from build123d import *
from build123d.topology import SkipClean

# Parameters (mm, degrees)
SKETCH1_R                      = 10.75
SKETCH1_R_2                    = 1.25
BOSS_EXTRUDE1_DEPTH            = 12
SKETCH14_R                     = 3.25
CUT_EXTRUDE3_DEPTH             = 2.3
CBORE_FOR_M3_SHCS2_D           = 3.4
CBORE_FOR_M3_SHCS2_CBORE_D     = 6.5
CBORE_FOR_M3_SHCS2_CBORE_DEPTH = 3
SKETCH3_R                      = 9.965776233
BOSS_EXTRUDE2_DEPTH            = 20
CUT_EXTRUDE2_REACH             = 37.428
CUT_EXTRUDE1_DEPTH             = 26.122201337
CUT_EXTRUDE1_DEPTH_BACK        = 2
SKETCH2_R                      = 3
SKETCH8_W                      = 1.35255
SKETCH8_H                      = 9.965776233
MOVE_START                     = 5.3
MOVE_FACE1_DEPTH               = 26.7
FILLET1_R                      = 10
CUT_EXTRUDE4_DEPTH             = 36.427743517
CUT_EXTRUDE4_DEPTH_BACK        = 36.427743517
SKETCH15_W                     = 19.931552466
SKETCH15_H                     = 6.64745


# Read off the part's stored shape, not the designer's step: Move Face1
with BuildPart() as part:
    # Sketch1 → Boss-Extrude1 (new body)
    with BuildSketch(Plane(origin=(0, 0, 0), x_dir=(1, 0, 0), z_dir=(0, 1, 0))):
        with Locations(Location((0, 0, 0), (0, 0, 270))):
            Circle(SKETCH1_R)
        with Locations(Location((-5.656854249, 5.656854249, 0), (0, 0, 270))):
            Circle(SKETCH1_R_2, mode=Mode.SUBTRACT)
        with Locations(Location((5.656854249, 5.656854249, 0), (0, 0, 270))):
            Circle(SKETCH1_R_2, mode=Mode.SUBTRACT)
        with Locations(Location((5.656854249, -5.656854249, 0), (0, 0, 270))):
            Circle(SKETCH1_R_2, mode=Mode.SUBTRACT)
        with Locations(Location((-5.656854249, -5.656854249, 0), (0, 0, 270))):
            Circle(SKETCH1_R_2, mode=Mode.SUBTRACT)
    extrude(amount=BOSS_EXTRUDE1_DEPTH)

    # Sketch14 → Cut-Extrude3 (cut)
    with BuildSketch(Plane.XZ):
        with Locations(Location((0, 0, 0), (0, 0, 270))):
            Circle(SKETCH14_R)
    extrude(amount=-CUT_EXTRUDE3_DEPTH, mode=Mode.SUBTRACT)

    # CBORE for M3 SHCS2 (through all)
    with Locations(Plane(origin=(0, 2.3, 0), x_dir=(-1, 0, 0), z_dir=(0, -1, 0))):
        with Locations((0, 0)):
            CounterBoreHole(CBORE_FOR_M3_SHCS2_D / 2, CBORE_FOR_M3_SHCS2_CBORE_D / 2, CBORE_FOR_M3_SHCS2_CBORE_DEPTH)

    # Sketch3 → Boss-Extrude2 (add)
    with BuildSketch(Plane(origin=(0, 12, 0), x_dir=(1, 0, 0), z_dir=(0, 1, 0))):
        with Locations(Location((0, 0, 0), (0, 0, 270))):
            Circle(SKETCH3_R)
    extrude(amount=BOSS_EXTRUDE2_DEPTH)

    # Sketch5 → Cut-Extrude2 (cut, up to next)
    with BuildSketch(Plane(origin=(0, 32, 0), x_dir=(1, 0, 0), z_dir=(0, 1, 0)), mode=Mode.PRIVATE) as cut_extrude2_sk1:
        with BuildLine():
            Line((-1.905, -2.54), (1.905, -2.54))
            ThreePointArc((1.905, -2.54), (0, 3.175), (-1.905, -2.54))
        make_face()
    cut_extrude2_tool1 = extrude(cut_extrude2_sk1.sketch, amount=-CUT_EXTRUDE2_REACH, mode=Mode.PRIVATE) & part.part
    add(cut_extrude2_tool1.solids().sort_by_distance((0, 32, -0.153521))[0], mode=Mode.SUBTRACT)

    # Sketch2 → Cut-Extrude1 (cut, two sides: drawn at the far end of the back side and taken through both)
    with BuildSketch(Plane(origin=(0, 12, 0), x_dir=(1, 0, 0), z_dir=(0, 1, 0)).offset(-CUT_EXTRUDE1_DEPTH_BACK)):
        with Locations((-5.656854249, 5.656854249)):
            Circle(SKETCH2_R)
        with Locations((5.656854249, 5.656854249)):
            Circle(SKETCH2_R)
        with Locations((5.656854249, -5.656854249)):
            Circle(SKETCH2_R)
        with Locations((-5.656854249, -5.656854249)):
            Circle(SKETCH2_R)
    extrude(amount=CUT_EXTRUDE1_DEPTH + CUT_EXTRUDE1_DEPTH_BACK, mode=Mode.SUBTRACT)

    # Sketch8 → Tap Drill for M3x0.5 Tap1 (revolve, cut)
    with BuildSketch(Plane(origin=(0, 22, 0), x_dir=(0, 1, 0), z_dir=(1, 0, 0))):
        with Locations((0.676275, 4.982888117)):
            Rectangle(SKETCH8_W, SKETCH8_H)
    revolve(axis=Axis((0, 22, -6.35), (0, 0, 1)), mode=Mode.SUBTRACT)

    # Move Face1 outline → Move Face1 (cut)
    with BuildSketch(Plane(origin=(0, 0, 0), x_dir=(1, 0, 0), z_dir=(0, 1, 0)).offset(MOVE_START)):
        with BuildLine():
            Line((-1.970539266, -2.74), (1.970539266, -2.74))
            ThreePointArc((1.970539266, -2.74), (0, 3.375), (-1.970539266, -2.74))
        make_face()
        with BuildLine():
            ThreePointArc((-1.905, -2.54), (0, 3.175), (1.905, -2.54))
            Line((1.905, -2.54), (-1.905, -2.54))
        make_face(mode=Mode.SUBTRACT)
    extrude(amount=MOVE_FACE1_DEPTH, mode=Mode.SUBTRACT)

    # Fillet1
    # the kernel refuses this fillet: 10 mm, written as the material it adds along each edge
    with BuildSketch(Plane(origin=(0, 12, 0), x_dir=(0.9978298678102888, 0, -0.06584493075174137), z_dir=(0.06584493075174137, 0, 0.9978298678102888))) as fillet1_piece_1_section:
        with BuildLine():
            CenterArc((19.965776233, 3.881941321), FILLET1_R, 180, 22.842179606)
            Line((9.965776233, 3.881941321), (9.765776233, 3.881941321))
            Line((9.765776233, 3.881941321), (9.765776233, 0))
            Line((9.765776233, 0), (9.965776233, -0.2))
            ThreePointArc((9.965776233, -0.2), (10.357888117, -0.2), (10.565684475, -0.077638826))
            Line((10.565684475, -0.077638826), (10.75, 0))
        make_face()
    fillet1_piece_1 = revolve(axis=Axis((0, 12, 0), (0, 1, 0)), revolution_arc=172.449263909, mode=Mode.PRIVATE)
    fillet1_piece_1 = fillet1_piece_1 - Plane(origin=(-5.656854249, 13.230633789, -5.656854249), x_dir=(1, 0, 0), z_dir=(0, 1, 0)) * Cylinder(3, 44, mode=Mode.PRIVATE)
    fillet1_piece_1 = fillet1_piece_1 - Plane(origin=(5.656854249, 13.230633789, -5.656854249), x_dir=(1, 0, 0), z_dir=(0, 1, 0)) * Cylinder(3, 44, mode=Mode.PRIVATE)
    add(fillet1_piece_1)
    with BuildSketch(Plane(origin=(0, 12, 0), x_dir=(0.06584493075180471, 0, 0.9978298678102845), z_dir=(-0.9978298678102845, 0, 0.06584493075180471))) as fillet1_piece_2_section:
        with BuildLine():
            CenterArc((19.965776233, 3.881941321), FILLET1_R, 180, 22.842179606)
            Line((9.965776233, 3.881941321), (9.765776233, 3.881941321))
            Line((9.765776233, 3.881941321), (9.765776233, 0))
            Line((9.765776233, 0), (9.965776233, -0.2))
            ThreePointArc((9.965776233, -0.2), (10.357888116, -0.2), (10.565684475, -0.077638826))
            Line((10.565684475, -0.077638826), (10.75, 0))
        make_face()
    fillet1_piece_2 = revolve(axis=Axis((0, 12, 0), (0, 1, 0)), revolution_arc=172.449263909, mode=Mode.PRIVATE)
    fillet1_piece_2 = fillet1_piece_2 - Plane(origin=(5.656854249, 13.23063377, 5.656854249), x_dir=(1, 0, 0), z_dir=(0, 1, 0)) * Cylinder(3, 43, mode=Mode.PRIVATE)
    fillet1_piece_2 = fillet1_piece_2 - Plane(origin=(5.656854249, 13.23063377, -5.656854249), x_dir=(1, 0, 0), z_dir=(0, 1, 0)) * Cylinder(3, 43, mode=Mode.PRIVATE)
    add(fillet1_piece_2)
    with BuildSketch(Plane(origin=(0, 12, 0), x_dir=(0.9978298678102888, 0, 0.0658449307517424), z_dir=(0.0658449307517424, 0, -0.9978298678102888))) as fillet1_piece_3_section:
        with BuildLine():
            CenterArc((19.965776233, -3.881941321), FILLET1_R, 157.157820394, 22.842179606)
            Line((9.965776233, -3.881941321), (9.765776233, -3.881941321))
            Line((9.765776233, -3.881941321), (9.765776233, 0))
            Line((9.765776233, 0), (9.965776233, 0.2))
            ThreePointArc((9.965776233, 0.2), (10.357888116, 0.2), (10.565684475, 0.077638826))
            Line((10.565684475, 0.077638826), (10.75, 0))
        make_face()
    fillet1_piece_3 = revolve(axis=Axis((0, 12, 0), (0, -1, 0)), revolution_arc=172.449263909, mode=Mode.PRIVATE)
    fillet1_piece_3 = fillet1_piece_3 - Plane(origin=(5.656854249, 13.230633816, 5.656854249), x_dir=(1, 0, 0), z_dir=(0, 1, 0)) * Cylinder(3, 44, mode=Mode.PRIVATE)
    fillet1_piece_3 = fillet1_piece_3 - Plane(origin=(-5.656854249, 13.230633816, 5.656854249), x_dir=(1, 0, 0), z_dir=(0, 1, 0)) * Cylinder(3, 44, mode=Mode.PRIVATE)
    add(fillet1_piece_3)
    with BuildSketch(Plane(origin=(0, 12, 0), x_dir=(-0.06584493075180468, 0, -0.9978298678102845), z_dir=(0.9978298678102845, 0, -0.06584493075180468))) as fillet1_piece_4_section:
        with BuildLine():
            CenterArc((19.965776233, 3.881941321), FILLET1_R, 180, 22.842179606)
            Line((9.965776233, 3.881941321), (9.765776233, 3.881941321))
            Line((9.765776233, 3.881941321), (9.765776233, 0))
            Line((9.765776233, 0), (9.965776233, -0.2))
            ThreePointArc((9.965776233, -0.2), (10.357888116, -0.2), (10.565684475, -0.077638826))
            Line((10.565684475, -0.077638826), (10.75, 0))
        make_face()
    fillet1_piece_4 = revolve(axis=Axis((0, 12, 0), (0, 1, 0)), revolution_arc=172.449263909, mode=Mode.PRIVATE)
    fillet1_piece_4 = fillet1_piece_4 - Plane(origin=(-5.656854249, 13.23063377, 5.656854249), x_dir=(1, 0, 0), z_dir=(0, 1, 0)) * Cylinder(3, 44, mode=Mode.PRIVATE)
    fillet1_piece_4 = fillet1_piece_4 - Plane(origin=(-5.656854249, 13.23063377, -5.656854249), x_dir=(1, 0, 0), z_dir=(0, 1, 0)) * Cylinder(3, 44, mode=Mode.PRIVATE)
    add(fillet1_piece_4)

    # Sketch15 → Cut-Extrude4 (cut, two sides: drawn at the far end of the back side and taken through both)
    with SkipClean():  # the faces are left unmerged after this step: merging them gives an invalid solid
        with BuildSketch(Plane.XY.offset(-CUT_EXTRUDE4_DEPTH_BACK)):
            with Locations((0, 28.676275)):
                Rectangle(SKETCH15_W, SKETCH15_H)
        extrude(amount=CUT_EXTRUDE4_DEPTH + CUT_EXTRUDE4_DEPTH_BACK, mode=Mode.SUBTRACT)


solid = part.part
Design review of the part built by this model. Coordinates are the model's own, in mm. A direction names the side the tool comes from. Round coordinates to 2 decimals unless told otherwise and drop trailing zeros. Order: outer loops, then holes, each group sorted by start corner. A loop starts at its lowest first (then second) coordinate and runs counter-clockwise, first axis right, second up. Notation, with made-up numbers: M 4.5,23.25 L 33.5,23.25 A23 cw 33.5,50.25 Z; hole C 30,3.5 d3. An arc over 180 degrees is marked long. Answer as CSV lines item,"result". Start each with the question number.
1) Wall thickness on line 1 along Z through (x, y) = (-3.75, 19); line 2 along X through (y, z) = (13.5, -5.25); line 3 along Z through (x, y) = (-4.75, 9): over which ranges is each line inside the solid? List them lowest first. Write a range as [from, to].
2) The part is to be moulded in two halves that separate along Y. For faces 1 (the face through (-5.6, 4.93, 4.41)), 2 (the face through (0.52, 23.25, 6.4)), 3 (the face through (3, 0, 2)), 4 (the face through (-4, 10, 6)), say which applies: +Y half, -Y half, draft (parallel to the pull), parting line (faces both ways), or undercut.
3) Add section A-A (y = 17). Give the boundary of the cut face in (x, z) (3 decimals).
4) Tool access review of faces 5 (the face through (-3.616, 17.569, -3.458)), 6 (the face through (-9.966, 20.551, -0.074)), 7 (the face through (0.074, 20.551, -9.966)), 8 (the face through (-0.074, 19.499, 9.966)), 9 (the face through (9.966, 20.551, 0.074)): name each direction out of +Z, -Z, +X, -X, +Y, -Y from which nothing blocks a thin tool from reaching the whole face with its end or side.
5) Add section B-B (z = 7.25). Give the boundary of the cut face in (x, y), then the cut area to 3 significant figures.
6) For pin 1 Ø8 at (x, y) = (7.5, 8.5) entering from +Z; pin 2 Ø3 at (x, z) = (-5.66, -5.66) entering from +Y; pin 3 Ø8 at (x, y) = (0, 14) entering from -Z; pin 4 Ø1.5 at (x, y) = (-7, 20.5) entering from +Z, all flat-tipped, find the tip position at first contact; note any pin that passes through.
7) Add section D-D (y = 21.25). Give the boundary of the cut face in (x, z) (3 decimals).
8) Add section C-C (y = 8.5). Give the boundary of the cut face in (x, z) (3 decimals), then the cut area to 3 significant figures.
Resolved:
1,line 1,"[-9.23, -7.97], [-3.34, 3.34], [7.97, 9.23]"
1,line 2,"[-8.81, -8.63], [-2.68, 2.68], [8.63, 8.81]"
1,line 3,"[-9.64, -6.52], [-4.8, 4.8], [6.52, 9.64]"
2,face 1,"draft"
2,face 2,"undercut"
2,face 3,"-Y half"
2,face 4,"+Y half"
3,outline,"M -8.594,-5.046 A3 cw long -5.046,-8.594 A9.966 ccw 5.046,-8.594 A3 cw long 8.594,-5.046 A9.966 ccw 8.594,5.046 A3 cw long 5.046,8.594 A9.966 ccw -5.046,8.594 A3 cw long -8.594,5.046 A9.966 ccw Z; hole M -1.971,2.74 A3.375 ccw long 1.971,2.74 Z"
4,face 5,"+Y"
4,face 6,"-X, +Y"
4,face 7,"-Z, +Y"
4,face 8,"+Z, +Y"
4,face 9,"+X, +Y"
5,outline,"M -7.94,0 L 7.94,0 L 7.94,10 L 3.11,10 L 3.11,25.35 L -3.11,25.35 L -3.11,10 L -7.94,10 Z; hole C 0,22 d2.71"
5,area,"249 mm^2"
6,pin 1,"z = 10.16"
6,pin 2,"y = 10"
6,pin 3,"z = -10.75"
6,pin 4,"z = 3.51"
7,outline,"M -8.594,-5.046 A3 cw long -5.046,-8.594 A9.966 ccw 5.046,-8.594 A3 cw long 8.594,-5.046 A9.966 ccw 8.594,5.046 A3 cw long 5.046,8.594 A9.966 ccw 1.126,9.902 L 1.126,2.74 L 1.971,2.74 A3.375 cw long -1.971,2.74 L -1.126,2.74 L -1.126,9.902 A9.966 ccw -5.046,8.594 A3 cw long -8.594,5.046 A9.966 ccw Z"
8,outline,"C 0,0 d21.5; hole C -5.657,-5.657 d2.5; hole C -5.657,5.657 d2.5; hole M -1.971,2.74 A3.375 ccw long 1.971,2.74 Z; hole C 5.657,-5.657 d2.5; hole C 5.657,5.657 d2.5"
8,area,"309 mm^2"
